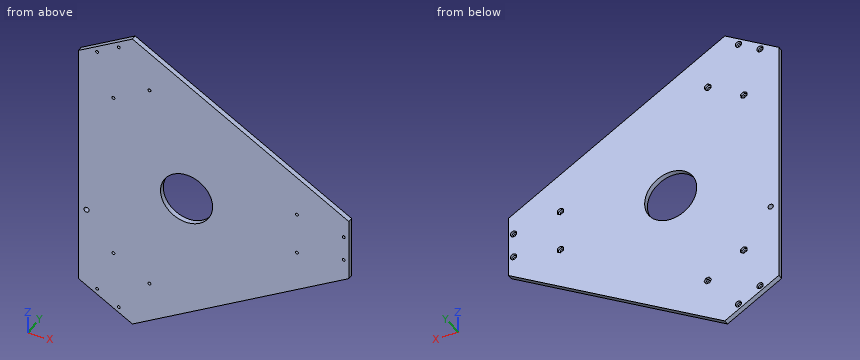
Autodesk Inventor part; units mm, degrees
ref_plane "YZ Plane" through (0, 0, 0) normal (1, 0, 0) x (0, 1, 0)
ref_plane "XZ Plane" through (0, 0, 0) normal (0, 1, 0) x (-1, 0, 0)
ref_plane "XY Plane" through (0, 0, 0) normal (0, 0, 1) x (1, 0, 0)
sketch "Sketch1" plane through (0, 0, 0) normal (0, 1, 0) x (-1, 0, 0)
  line L0 (-259.8076, 150) -> (-259.8076, 90)
  line L1 (-259.8076, 90) -> (-51.9615, -30)
  line L2 (-51.9615, -30) -> (0, 0)
  line L3 (0, 0) -> (0, 240)
  line L4 (0, 240) -> (-51.9615, 270)
  line L5 (-51.9615, 270) -> (-259.8076, 150)
  dimension "d0" = 120
  dimension "d1" = 120
  dimension "d2" = 120
  dimension "d4" = 120
  dimension "d5" = 120
  dimension "d6" = 60
  dimension "d7" = 120
extrude "Extrusion1" add sketch "Sketch1" along normal blind 5
sketch "Sketch2" plane through (0, 5, 0) normal (0, 1, 0) x (1, 0, 0)
  line L0 (254.8076, -108) -> (254.8076, -132)
  line L1 (259.8076, -150) -> (259.8076, -90)
  line L2 (259.8076, -90) -> (51.9615, 30)
  line L3 (51.9615, -270) -> (259.8076, -150)
  line L4 (209.8076, -108) -> (209.8076, -132)
  line L5 (209.8076, -108) -> (209.8076, -100)
  line L6 (209.8076, -144.7569) -> (209.8076, -140)
  point P0 (0, 0)
  dimension "d10" = 24
  dimension "d11" = 5
  dimension "d12" = 18
  dimension "d31" = 18.0885
  dimension "d32" = 18.0885
  dimension "d33" = 18
  dimension "d44" = 45
  dimension "d45" = 0
  dimension "d47" = 40.5885
  dimension "d51" = 8
  dimension "d52" = 8
hole "Hole1" at (209.8076, 5, 100) at (209.8076, 5, 140) at (254.8076, 5, 108) at (254.8076, 5, 132) direction (0, -1, 0) diameter 2.8 end through all
sketch "Sketch3" plane through (0, 5, 0) normal (0, 1, 0) x (1, 0, 0)
  line L0 (18.088, 4.6696) -> (38.8735, 16.6701)
  line L1 (51.9615, 30) -> (0, 0)
  line L2 (0, 0) -> (0, -240)
  line L3 (259.8076, -90) -> (51.9615, 30)
  line L4 (47.516, -30.3017) -> (68.3015, -18.3011)
  line L5 (68.3015, -18.3011) -> (68.3015, -18.3011)
  line L6 (47.516, -30.3017) -> (33.66, -38.3014)
  dimension "d20" = 5
  dimension "d22" = 18.088
  dimension "d23" = 18.088
  dimension "d46" = 45
  dimension "d48" = 33.66
  dimension "d53" = 33.66
  dimension "d89" = 33.66
hole "Hole2" at (68.3015, 5, 18.3011) at (33.66, 5, 38.3014) at (18.088, 5, -4.6696) at (38.8735, 5, -16.6701) direction (0, -1, 0) diameter 2.8 end through all
sketch "Sketch4" plane through (0, 5, 0) normal (0, 1, 0) x (1, 0, 0)
  line L0 (18.088, -244.6696) -> (38.8735, -256.6701)
  line L1 (0, -240) -> (51.9615, -270)
  line L2 (51.9615, -270) -> (259.8076, -150)
  line L3 (0, 0) -> (0, -240)
  line L4 (47.516, -209.6983) -> (68.3015, -221.6989)
  line L5 (68.3015, -221.6989) -> (68.3015, -221.6989)
  line L6 (47.516, -209.6983) -> (33.66, -201.6986)
  dimension "d34" = 5
  dimension "d35" = 18.088
  dimension "d36" = 18.088
  dimension "d49" = 45
  dimension "d50" = 33.66
  dimension "d56" = 33.66
  dimension "d90" = 33.66
hole "Hole3" at (68.3015, 5, 221.6989) at (33.66, 5, 201.6986) at (18.088, 5, 244.6696) at (38.8735, 5, 256.6701) direction (0, -1, 0) diameter 2.8 end through all
sketch "Sketch5" plane through (0, 5, 0) normal (0, 1, 0) x (1, 0, 0)
  circle A0 centre (103.923, -120) radius 25
  line L0 (0, 0) -> (0, -240)
  line L1 (259.8076, -90) -> (51.9615, 30)
  line L2 (51.9615, 30) -> (0, 0)
  line L3 (25.9808, 15) -> (155.8846, -210)
  line L4 (51.9615, -270) -> (259.8076, -150)
  line L5 (51.9615, 30) -> (0, 0)
  line L6 (0, 0) -> (0, -240)
  line L7 (0, -120) -> (259.8076, -120)
  line L8 (259.8076, -150) -> (259.8076, -90)
  line L9 (0, -240) -> (51.9615, -270)
  line L10 (25.9808, -255) -> (155.8846, -30)
  dimension "d57" = 50
  dimension "d60" = 0
  dimension "d61" = 0
extrude "Extrusion2" cut sketch "Sketch5" against normal through all contours L7 L10 A0 | A0 L3 L7 | L10 L3 A0 | A0 L10 L3 | L7 A0 L3 | L10 A0 L7
sketch "Sketch6" plane through (0, 5, 0) normal (0, 1, 0) x (1, 0, 0)
  circle A0 centre (103.923, -120) radius 25
  circle A1 centre (18.088, -244.6696) radius 1.4
  circle A2 centre (68.3015, -221.6989) radius 1.4
  circle A3 centre (33.66, -201.6986) radius 1.4
  circle A4 centre (38.8735, -256.6701) radius 1.4
  circle A5 centre (18.088, 4.6696) radius 1.4
  circle A6 centre (68.3015, -18.3011) radius 1.4
  circle A7 centre (33.66, -38.3014) radius 1.4
  circle A8 centre (38.8735, 16.6701) radius 1.4
  circle A9 centre (254.8076, -108) radius 1.4
  circle A10 centre (209.8076, -100) radius 1.4
  circle A11 centre (209.8076, -140) radius 1.4
  circle A12 centre (254.8076, -132) radius 1.4
  line L0 (259.8076, -90) -> (51.9615, 30)
  line L1 (51.9615, 30) -> (0, 0)
  line L2 (0, 0) -> (0, -240)
  line L3 (0, -240) -> (51.9615, -270)
  line L4 (51.9615, -270) -> (259.8076, -150)
  line L5 (259.8076, -150) -> (259.8076, -90)
  line L6 (36.3641, -199.5334) -> (36.8871, -202.9578)
  line L7 (36.8871, -202.9578) -> (34.183, -205.123)
  line L8 (34.183, -205.123) -> (30.9559, -203.8638)
  line L9 (30.9559, -203.8638) -> (30.4329, -200.4394)
  line L10 (30.4329, -200.4394) -> (33.137, -198.2742)
  line L11 (33.137, -198.2742) -> (36.3641, -199.5334)
  circle A13 centre (68.3015, -221.6989) radius 1.4
  line L12 (67.8588, -218.2632) -> (71.0556, -219.5976)
  line L13 (71.0556, -219.5976) -> (71.4983, -223.0333)
  line L14 (71.4983, -223.0333) -> (68.7442, -225.1346)
  line L15 (68.7442, -225.1346) -> (65.5475, -223.8001)
  line L16 (65.5475, -223.8001) -> (65.1048, -220.3644)
  line L17 (65.1048, -220.3644) -> (67.8588, -218.2632)
  circle A14 centre (209.8076, -140) radius 1.4
  line L18 (212.8076, -138.2679) -> (212.8076, -141.7321)
  line L19 (212.8076, -141.7321) -> (209.8076, -143.4641)
  line L20 (209.8076, -143.4641) -> (206.8076, -141.7321)
  line L21 (206.8076, -141.7321) -> (206.8076, -138.2679)
  line L22 (206.8076, -138.2679) -> (209.8076, -136.5359)
  line L23 (209.8076, -136.5359) -> (212.8076, -138.2679)
  line L24 (206.8076, -98.2679) -> (209.8076, -96.5359)
  line L25 (209.8076, -96.5359) -> (212.8076, -98.2679)
  line L26 (212.8076, -98.2679) -> (212.8076, -101.7321)
  line L27 (212.8076, -101.7321) -> (209.8076, -103.4641)
  line L28 (209.8076, -103.4641) -> (206.8076, -101.7321)
  line L29 (206.8076, -101.7321) -> (206.8076, -98.2679)
  circle A15 centre (68.3015, -18.3011) radius 1.4
  line L30 (69.9304, -15.2439) -> (71.7636, -18.1831)
  line L31 (71.7636, -18.1831) -> (70.1348, -21.2404)
  line L32 (70.1348, -21.2404) -> (66.6727, -21.3584)
  line L33 (66.6727, -21.3584) -> (64.8394, -18.4191)
  line L34 (64.8394, -18.4191) -> (66.4683, -15.3619)
  line L35 (66.4683, -15.3619) -> (69.9304, -15.2439)
  circle A16 centre (33.66, -38.3014) radius 1.4
  line L36 (33.66, -34.8373) -> (36.66, -36.5694)
  line L37 (36.66, -36.5694) -> (36.66, -40.0335)
  line L38 (36.66, -40.0335) -> (33.66, -41.7655)
  line L39 (33.66, -41.7655) -> (30.66, -40.0335)
  line L40 (30.66, -40.0335) -> (30.66, -36.5694)
  line L41 (30.66, -36.5694) -> (33.66, -34.8373)
  line L42 (0, 0) -> (0, -240)
  line L43 (51.9615, -270) -> (259.8076, -150)
  line L44 (259.8076, -90) -> (51.9615, 30)
  circle A17 centre (18.088, -244.6696) radius 3
  circle A18 centre (38.8735, -256.6701) radius 3
  circle A19 centre (18.088, 4.6696) radius 3
  circle A20 centre (38.8735, 16.6701) radius 3
  circle A21 centre (254.8076, -108) radius 3
  circle A22 centre (254.8076, -132) radius 3
  dimension "d66" = 6
  dimension "d67" = 6
  dimension "d68" = 6
  dimension "d71" = 6
  dimension "d72" = 6
  dimension "d73" = 6
  dimension "d78" = 6
  dimension "d79" = 6
  dimension "d80" = 6
  dimension "d81" = 6
  dimension "d82" = 6
  dimension "d83" = 6
extrude "Extrusion3" cut sketch "Sketch6" against normal blind 2.5 contours A1 | A4 | A5 | A6 | A8 | A9 | A10 | A11 | A12 | L6 L7 L8 L9 L10 L11 | L12 L13 L14 L15 L16 L17 | L18 L19 L20 L21 L22 L23 | L24 L25 L26 L27 L28 L29 | L30 L31 L32 L33 L34 L35 | L36 L37 L38 L39 L40 L41 | A17 | A18 | A19 | A20 | A21 | A22
sketch "Sketch7" plane through (0, 5, 0) normal (0, 1, 0) x (1, 0, 0)
  circle A0 centre (7.9, -75) radius 2.5
  line L0 (0, 0) -> (0, -240)
  dimension "d84" = 75
  dimension "d85" = 5
  dimension "d88" = 7.9
extrude "Extrusion4" cut sketch "Sketch7" against normal through all
properties part number "lep_felso" material "Wood (Birch)"
CAD build for the part. Positions are in the model's coordinates, mm. Give positions to 0.01 mm unless a question says otherwise; leave off trailing zeros. Write each loop counter-clockwise with the first axis right and the second up, starting at its lowest first coordinate (ties: lowest second). Pieces come first, ordered by that corner, then holes. Notation, with made-up numbers: (33, 37) - (77, 37) arc R15 ccw to (77, 48) - close; hole circle Ø6 at (3.25, 51). An arc over 180 degrees is marked (long way). Put each result on its own line as item: value.
(1) Saw through at B-B (x = 99). List the corners of the cut face in (y, z), then the cut area to 3 significant figures.
Working result:
outline: (0, -2.84) - (5, -2.84) - (5, 95.49) - (0, 95.49) - close; (0, 144.51) - (5, 144.51) - (5, 242.84) - (0, 242.84) - close
area: 983 mm^2
(2) Drop flat-ended pins along their axis: pin 1 Ø3.5 at (x, z) = (18.09, -4.67) entering from +Y; pin 2 Ø1 at (x, y) = (225.5, 4) entering from +Z; pin 3 Ø2 at (y, z) = (4, 39) entering from +X. Give the stop position or say it passes through.
Working result:
pin 1: y = 2.5
pin 2: z = 170.1
pin 3: x = 173.21
(3) Wall check: L1, parallel to X at y = 1.35, z = 108; L2, parallel to X at y = 4.3, z = 108; L3, parallel to X at y = 0.4, z = 76.5. Give the ranges that are in metal, low to high.
Working result:
L1: 0 to 81.99, 125.85 to 253.41, 256.21 to 259.81
L2: 0 to 81.99, 125.85 to 251.81, 257.81 to 259.81
L3: 0 to 5.9, 9.9 to 236.42
(4) Saw through at D-D (x = 46). List the corners of the cut face in (y, z).
Working result:
outline: (0, -26.56) - (5, -26.56) - (5, 266.56) - (0, 266.56) - close
(5) Saw through at C-C (y = 0.9). Count the separate pieces of the cut face and the enclosed holes in it, then the cut area to 3 significant figures.
Working result:
separate pieces: 1
enclosed holes: 14
area: 49,400 mm^2
(6) Saw through at A-A (z = 120). List the corners of the cut face in (x, y).
Working result:
outline: (0, 0) - (78.92, 0) - (78.92, 5) - (0, 5) - close; (128.92, 0) - (259.81, 0) - (259.81, 5) - (128.92, 5) - close
